from build123d import *

# Parameters (mm, degrees)
F0_R     = 5
F1_DEPTH = 3
F0_W     = 4.25
F0_H     = 4.3
F2_DEPTH = 10
F3_R     = 6.25
F3_R_2   = 5
F3_W     = 4.25
F3_H     = 4.3
F4_DEPTH = 2


with BuildPart() as f1:
    # F0 (on Top) → F1 (new body)
    with BuildSketch(Plane.XY):
        with BuildLine():
            ThreePointArc((1, -8.944272), (6.708204, -6), (9, 0))
            ThreePointArc((9, 0), (-6, 6.708204), (-1, -8.944272))
            ThreePointArc((-1, -8.944272), (0, -9), (1, -8.944272))
        make_face()
        Circle(F0_R, mode=Mode.SUBTRACT)
    extrude(amount=F1_DEPTH)

    # F0 (on Top) → F2 (join)
    with BuildSketch(Plane.XY):
        Circle(F0_R)
        Rectangle(F0_W, F0_H, mode=Mode.SUBTRACT)
    extrude(amount=F2_DEPTH)

    # F3 (on face) → F4 (join)
    with BuildSketch(Plane.XY.offset(10)):
        Circle(F3_R)
        Circle(F3_R_2, mode=Mode.SUBTRACT)
        Circle(F3_R_2)
        Rectangle(F3_W, F3_H, mode=Mode.SUBTRACT)
    extrude(amount=-F4_DEPTH)


solid = f1.part
CAD build for the part. Positions are in the model's coordinates, mm. A direction names the side the tool comes from. Round coordinates to 2 decimals unless told otherwise and drop trailing zeros. Loops run counter-clockwise (first coordinate to the right, second up) from the corner with the lowest first, then second, coordinate; pieces in that order, holes last. Notation, with made-up numbers: (12.5, 31) - (53.5, 31) arc R34 cw to (53.5, 61) - close; hole circle Ø6 at (-18, 2.5). An arc over 180 degrees is marked (long way). Put each result on its own line as item: value.
1. Slice it at C-C on y = 5.5. List the corners of the cut face in (x, z), and give its area (3 significant figures).
Geometry check:
outline: (-7.12, 0) - (7.12, 0) - (7.12, 3) - (-7.12, 3) - close; (-2.97, 8) - (2.97, 8) - (2.97, 10) - (-2.97, 10) - close
area: 54.6 mm²
2. Slice it at A-A on x = 0. List the corners of the cut face in (y, z), and give its area (3 significant figures).
Geometry check:
outline: (-9, 0) - (-2.15, 0) - (-2.15, 10) - (-6.25, 10) - (-6.25, 8) - (-5, 8) - (-5, 3) - (-9, 3) - close; (2.15, 0) - (9, 0) - (9, 3) - (5, 3) - (5, 8) - (6.25, 8) - (6.25, 10) - (2.15, 10) - close
area: 86.0 mm²
3. Pin check, flat tips, straight feed: P1, Ø4, axis at x = -6.5, z = 7, coming from the -Y side; P2, Ø4.5, axis at x = 1, z = 6, coming from the -Y side; P3, Ø1.5, axis at x = -3.5, z = 4.5, coming from the -Y side. Stop position of each tip, or through.
Geometry check:
P1: y = -4.04
P2: y = -6.25
P3: y = -4.18
4. Slice it at D-D on x = -2.75. List the corners of the cut face in (y, z).
Geometry check:
outline: (-8.57, 0) - (8.57, 0) - (8.57, 3) - (4.18, 3) - (4.18, 8) - (5.61, 8) - (5.61, 10) - (-5.61, 10) - (-5.61, 8) - (-4.18, 8) - (-4.18, 3) - (-8.57, 3) - close
5. Slice it at B-B on z = 7. List the corners of the cut face in (x, y) (3 decimals), and give its area (3 significant figures).
Geometry check:
outline: circle Ø10 at (0, 0); hole (-2.125, -2.15) - (2.125, -2.15) - (2.125, 2.15) - (-2.125, 2.15) - close
area: 60.3 mm²
6. 3-axis set-ups, long thin cutter, end or side, ignore diameter. For faces 5 (the flat face through (-2.125, 0, 5)), 6 (the flat face through (0, -3, 10)), 7 (the cylindrical face through (0, -9, 1)), 8 (the flat face through (2, 5, 8)), 9 (the cylindrical face through (5.96, 1.88, 9.01)): which of +Z, -Z, +X, -X, +Y, -Y reach the whole face in a straight line?
Geometry check:
face 5: +Z, -Z
face 6: +Z, +X, -X, +Y, -Y
face 7: +Z, -Z, -Y
face 8: none
face 9: +Z
7. Wall check: line 1 (Y direction, x = -0.25, z = 1.5); line 2 (X direction, y = 0.25, z = 8.25) (3 decimals); line 3 (Z direction, x = 1.75, y = 5.75). Give the ranges that are in metal, low to high.
Geometry check:
line 1: -9 to -2.15, 2.15 to 9
line 2: -6.245 to -2.125, 2.125 to 6.245
line 3: 0 to 3, 8 to 10
8. Two-plate mould, pull along X, no slides. Class faces 1 (the flat face through (2.125, 0, 5)), 2 (the cylindrical face through (-1.08, -4.88, 5.46)), 3 (the flat face through (0, 2.15, 5)), 4 (the flat face through (4, -4, 3)): released by +X, released by -X, zero draft, split by the parting line, or undercut.
Geometry check:
face 1: undercut
face 2: split by the parting line
face 3: undercut
face 4: zero draft
